Can you work these out from the model? Positions are in its coordinate system, mm. Face numbers are marked on the shaded views. A direction names the side the tool comes from. Coordinates: 2 decimals unless noted, no trailing zeros. Loops run counter-clockwise (first coordinate to the right, second up) from the corner with the lowest first, then second, coordinate; pieces in that order, holes last. Notation, with made-up numbers: (47.5, -30) -> (72.5, -30) arc R27 cw to (72.5, 9) -> close; hole circle Ø2 at (3, 14.25). An arc over 180 degrees is marked (long way). Use one line per item in the form item = value. Start each with the question number.
(1) Thinking about a two-plate mould opening in X: for the marked faces 1, 2, 3 and 4, which applies, released by +X, released by -X, zero draft, split by the parting line, or undercut?
(2) I'm going to push flat-ended pins straight in: pin 1 (1.5 mm diameter, centred on x = 2.5, z = 11.5, fed in from +Y); pin 2 (4 mm diameter, centred on x = -3.5, y = -4, fed in from +Z); pin 3 (6 mm diameter, centred on x = -3.5, z = 21, fed in from +Y). Where does each tip first touch, or does it pass through?
(3) I need wall thicknesses on line 1 (Z direction, x = -4, y = 0); line 2 (Z direction, x = -0.5, y = -1.5); line 3 (Y direction, x = 4, z = 4.5). Which ranges of each line are inside material? Lowest first, please. Write a range as [from, to].
(4) Imagine slicing it at D-D (y = 1.75). List the corners of the cut face in (x, z) for me, plus the area to 3 significant figures.
(5) Imagine slicing it at A-A (y = 0). List the corners of the cut face in (x, z) for me.
(6) Imagine slicing it at C-C (z = 17.75). List the corners of the cut face in (x, y) for me, plus the area to 3 significant figures.
(7) On a 3-axis mill with a long thin cutter (end or side, diameter ignored), from which of +Z, -Z, +X, -X, +Y, -Y can I reach the whole of each face in a straight line? I mean the marked faces 5 and 6. Say none if no direction works.
(8) Imagine slicing it at B-B (x = 2.75). List the corners of the cut face in (y, z) for me.
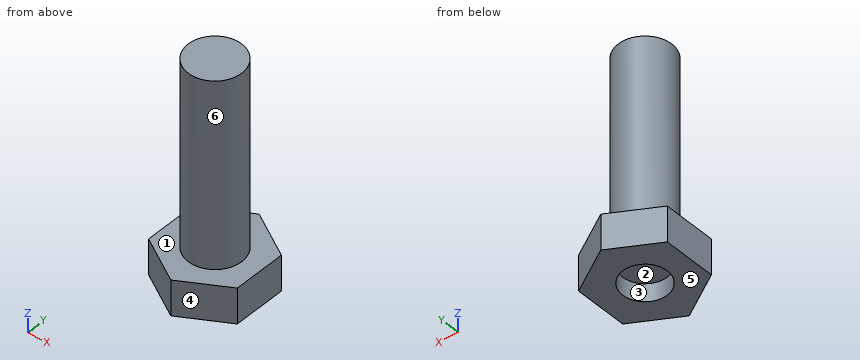
```python
from build123d import *

# Parameters (mm, degrees)
PAD007_DEPTH    = 4
SKETCH011_R     = 3
PAD008_DEPTH    = 21
SKETCH013_R     = 2.5
POCKET001_DEPTH = 2


with BuildPart() as part:
    # Sketch010 → Pad007 (new body)
    with BuildSketch(Plane.XY):
        Polygon((5, -2.886751), (5, 2.886751), (0, 5.773503), (-5, 2.886751), (-5, -2.886751), (0, -5.773503), align=None)
    extrude(amount=-PAD007_DEPTH)

    # Sketch011 → Pad008 (join)
    with BuildSketch(Plane.XY):
        Circle(SKETCH011_R)
    extrude(amount=PAD008_DEPTH)

    # Sketch013 → Pocket001 (cut)
    with BuildSketch(Plane.XY.offset(-4)):
        Circle(SKETCH013_R)
    extrude(amount=POCKET001_DEPTH, mode=Mode.SUBTRACT)


with BuildPart() as part_1:
    # Body007 placement: moved
    add(part.part.moved(Location((0, 0, 7))))


solid = part_1.part
```
Worked out:
q1.face_1 = zero draft
q1.face_2 = undercut
q1.face_3 = undercut
q1.face_4 = released by +X
q2.pin_1 = 2.44
q2.pin_2 = 7
q2.pin_3 = 2.96
q3.line_1 = [3, 7]
q3.line_2 = [5, 28]
q3.line_3 = [-3.46, 3.46]
q4.outline = (-5, 3) -> (-1.79, 3) -> (-1.79, 5) -> (1.79, 5) -> (1.79, 3) -> (5, 3) -> (5, 7) -> (2.44, 7) -> (2.44, 28) -> (-2.44, 28) -> (-2.44, 7) -> (-5, 7) -> close
q4.area = 135 mm2
q5.outline = (-5, 3) -> (-2.5, 3) -> (-2.5, 5) -> (2.5, 5) -> (2.5, 3) -> (5, 3) -> (5, 7) -> (3, 7) -> (3, 28) -> (-3, 28) -> (-3, 7) -> (-5, 7) -> close
q6.outline = circle Ø6 at (0, 0)
q6.area = 28.3 mm2
q7.face_5 = -Z, +X, -X, +Y, -Y
q7.face_6 = +Z
q8.outline = (-4.19, 3) -> (4.19, 3) -> (4.19, 7) -> (1.2, 7) -> (1.2, 28) -> (-1.2, 28) -> (-1.2, 7) -> (-4.19, 7) -> close
